```python
from build123d import *

# Parameters (mm, degrees)
SALIENTE_EXTRUIR1_DEPTH = 12.7
CROQUIS2_R              = 3
CORTAR_EXTRUIR1_DEPTH   = 3
CROQUIS3_R              = 10
CROQUIS3_R_2            = 2
CORTAR_EXTRUIR2_DEPTH   = 31
CROQUIS4_R              = 1.5
CORTAR_EXTRUIR3_DEPTH   = 31
CROQUIS5_R              = 4
CORTAR_EXTRUIR4_DEPTH   = 3
CROQUIS6_R              = 25.5
CORTAR_EXTRUIR5_DEPTH   = 2.55


with BuildPart() as part:
    # Croquis1 → Saliente-Extruir1 (new body)
    with BuildSketch(Plane.XY):
        with BuildLine():
            Line((10, 0), (90, 0))
            ThreePointArc((90, 0), (97.071067812, 2.928932188), (100, 10))
            Line((100, 10), (100, 90))
            ThreePointArc((100, 90), (97.071067812, 97.071067812), (90, 100))
            Line((90, 100), (10, 100))
            ThreePointArc((10, 100), (2.928932188, 97.071067812), (0, 90))
            Line((0, 90), (0, 10))
            ThreePointArc((0, 10), (2.928932188, 2.928932188), (10, 0))
        make_face()
    extrude(amount=SALIENTE_EXTRUIR1_DEPTH)

    # Croquis2 → Cortar-Extruir1 (cut)
    with BuildSketch(Plane.XY.offset(12.7)):
        with Locations((10, 88)):
            Circle(CROQUIS2_R)
        with Locations((10, 8)):
            Circle(CROQUIS2_R)
        with Locations((90, 88)):
            Circle(CROQUIS2_R)
        with Locations((90, 8)):
            Circle(CROQUIS2_R)
    extrude(amount=-CORTAR_EXTRUIR1_DEPTH, mode=Mode.SUBTRACT)

    # Croquis3 → Cortar-Extruir2 (cut)
    with BuildSketch(Plane.XY.offset(12.7)):
        with Locations((50, 50)):
            Circle(CROQUIS3_R)
        with Locations((25.125, 74.875)):
            Circle(CROQUIS3_R_2)
        with Locations((74.875, 74.875)):
            Circle(CROQUIS3_R_2)
        with Locations((25.125, 25.125)):
            Circle(CROQUIS3_R_2)
        with Locations((74.875, 25.125)):
            Circle(CROQUIS3_R_2)
    extrude(amount=-CORTAR_EXTRUIR2_DEPTH, mode=Mode.SUBTRACT)

    # Croquis4 → Cortar-Extruir3 (cut)
    with BuildSketch(Plane.XY.offset(9.7)):
        with Locations((10, 88)):
            Circle(CROQUIS4_R)
        with Locations((90, 88)):
            Circle(CROQUIS4_R)
        with Locations((90, 8)):
            Circle(CROQUIS4_R)
        with Locations((10, 8)):
            Circle(CROQUIS4_R)
    extrude(amount=-CORTAR_EXTRUIR3_DEPTH, mode=Mode.SUBTRACT)

    # Croquis5 → Cortar-Extruir4 (cut)
    with BuildSketch(Plane(origin=(0, 0, 0), x_dir=(-1, 0, 0), z_dir=(0, 0, -1))):
        with Locations((-74.875, 74.875)):
            Circle(CROQUIS5_R)
        with Locations((-25.125, 74.875)):
            Circle(CROQUIS5_R)
        with Locations((-25.125, 25.125)):
            Circle(CROQUIS5_R)
        with Locations((-74.875, 25.125)):
            Circle(CROQUIS5_R)
    extrude(amount=-CORTAR_EXTRUIR4_DEPTH, mode=Mode.SUBTRACT)

    # Croquis6 → Cortar-Extruir5 (cut)
    with BuildSketch(Plane.XY.offset(12.7)):
        with Locations((50, 50)):
            Circle(CROQUIS6_R)
    extrude(amount=-CORTAR_EXTRUIR5_DEPTH, mode=Mode.SUBTRACT)


solid = part.part
```
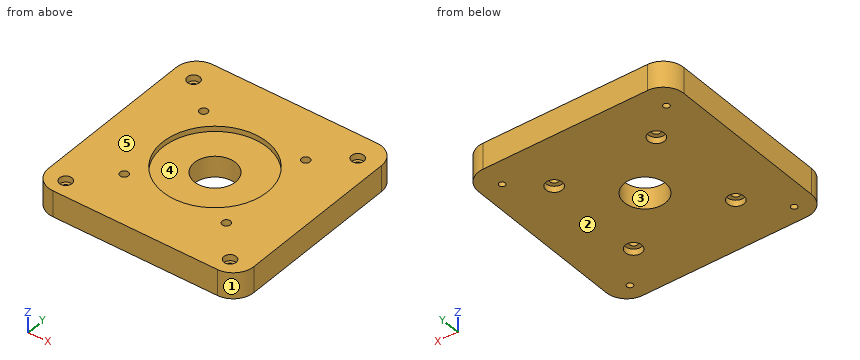
The listing builds one solid part. Answer for the finished solid, in the listing's coordinates (mm). Face numbers are marked on the shaded views. A direction names the side the tool comes from. Coordinates: 2 decimals unless noted, no trailing zeros. Write each loop counter-clockwise with the first axis right and the second up, starting at its lowest first coordinate (ties: lowest second). Pieces come first, ordered by that corner, then holes.
Q1. Section D-D, the plane z = 7 is taken. Give the number of separate pieces and of enclosed holes in the cut face, then the cut area to 3 significant figures.
Returned:
separate pieces: 1
enclosed holes: 9
area: 9,520 mm2
Q2. Section A-A, the plane y = 50 is taken. Write down the section's boundary in (x, z), then the cut area to 3 significant figures.
Returned:
outline: (0, 0) - (40, 0) - (40, 10.15) - (24.5, 10.15) - (24.5, 12.7) - (0, 12.7) - close; (60, 0) - (100, 0) - (100, 12.7) - (75.5, 12.7) - (75.5, 10.15) - (60, 10.15) - close
area: 937 mm2
Q3. The mould has two halves that part along X. Classify the marked faces 1, 2 and 3: released by +X, released by -X, zero draft, split by the parting line, or undercut.
Returned:
face 1: released by +X
face 2: zero draft
face 3: undercut
Q4. Given P1, Ø4, axis at x = 65, y = 87, coming from the -Z side; P2, Ø3.5, axis at x = 90, y = 88, coming from the +Z side; P3, Ø2.5, axis at x = 26.5, y = 27, coming from the -Z side, each flat-ended and moving along its own axis, determine where each tip first touches the part or whether it passes through.
Returned:
P1: stops at z = 0
P2: stops at z = 9.7
P3: stops at z = 3
Q5. Find the intervals of material crossed by line 1 along Y through (x, z) = (10, 3.5); line 2 along X through (y, z) = (88, 6.25); line 3 along X through (y, z) = (78.5, 1.25), in increasing order.
Returned:
line 1: y = 0 to 6.5, 9.5 to 86.5, 89.5 to 100
line 2: x = 0 to 8.5, 11.5 to 88.5, 91.5 to 100
line 3: x = 0 to 23.43, 26.82 to 73.18, 76.57 to 100
Q6. Which of the six approach directions +Z, -Z, +X, -X, +Y, -Y give full straight-line access (tool end or side, diameter ignored) to the marked faces 4 and 5?
Returned:
face 4: +Z
face 5: +Z, +X, -X, +Y, -Y
Q7. Section C-C, the plane y = 88 is taken. Write down the section's boundary in (x, z), then the cut area to 3 significant figures.
Returned:
outline: (0, 0) - (8.5, 0) - (8.5, 9.7) - (7, 9.7) - (7, 12.7) - (0, 12.7) - close; (11.5, 0) - (88.5, 0) - (88.5, 9.7) - (87, 9.7) - (87, 12.7) - (13, 12.7) - (13, 9.7) - (11.5, 9.7) - close; (91.5, 0) - (100, 0) - (100, 12.7) - (93, 12.7) - (93, 9.7) - (91.5, 9.7) - close
area: 1,180 mm2
